```python
from build123d import *

# Parameters (mm, degrees)
SKETCH_1_W           = 300
SKETCH_1_H           = 30
EXTRUDE_1_DEPTH      = 20
EXTRUDE_2_DEPTH      = 28
EXTRUDE_2_DEPTH_BACK = 328
SKETCH_3_R           = 4
CUT_EXTRUDE_1_DEPTH  = 182.614977356
SKETCH_3_3_R         = 6
SKETCH_3_3_R_2       = 4
CUT_EXTRUDE_2_DEPTH  = 182.614977356
SKETCH_3_4_R         = 13.5
SKETCH_3_4_R_2       = 13.25
SKETCH_3_4_R_3       = 6
CUT_EXTRUDE_3_DEPTH  = 182.614977356
SKETCH_3_5_R         = 2.4
CUT_EXTRUDE_4_DEPTH  = 4.5
SKETCH_3_6_R         = 2.4
CUT_EXTRUDE_5_DEPTH  = 5
SKETCH_9_W           = 8.22
SKETCH_9_H           = 5
CUT_EXTRUDE_6_DEPTH  = 182.295339172
CUT_EXTRUDE_7_REACH  = 183.615
SKETCH_11_R          = 2.55


with BuildPart() as part:
    # Sketch 1 → Extrude 1 (new body)
    with BuildSketch(Plane.XY):
        with Locations((0, 15)):
            Rectangle(SKETCH_1_W, SKETCH_1_H)
    extrude(amount=EXTRUDE_1_DEPTH)

    # Sketch 2 → Extrude 2 (add, two sides: drawn at the far end of the back side and taken through both)
    with BuildSketch(Plane.ZY.offset(150).offset(-EXTRUDE_2_DEPTH_BACK)):
        with BuildLine():
            Line((0, 20), (0, 10))
            ThreePointArc((0, 10), (5, 15), (0, 20))
        make_face()
    extrude(amount=EXTRUDE_2_DEPTH + EXTRUDE_2_DEPTH_BACK)

    # Sketch 3 → Cut-Extrude 1 (cut, through all)
    with BuildSketch(Plane(origin=(0, 0, 0), x_dir=(-1, 0, 0), z_dir=(0, 0, -1))):
        with Locations((0, 15)):
            Circle(SKETCH_3_R)
    extrude(amount=-CUT_EXTRUDE_1_DEPTH, mode=Mode.SUBTRACT)

    # Sketch 3_3 → Cut-Extrude 2 (cut, through all)
    with BuildSketch(Plane(origin=(0, 0, 0), x_dir=(-1, 0, 0), z_dir=(0, 0, -1))):
        with Locations((0, 15)):
            Circle(SKETCH_3_3_R)
        with Locations((0, 15)):
            Circle(SKETCH_3_3_R_2, mode=Mode.SUBTRACT)
    extrude(amount=-CUT_EXTRUDE_2_DEPTH, mode=Mode.SUBTRACT)

    # Sketch 3_4 → Cut-Extrude 3 (cut, through all)
    # profile 1 of 2: a face of its own
    with BuildSketch(Plane(origin=(0, 0, 0), x_dir=(-1, 0, 0), z_dir=(0, 0, -1))):
        with Locations((0, 15)):
            Circle(SKETCH_3_4_R)
        with Locations((0, 15)):
            Circle(SKETCH_3_4_R_2, mode=Mode.SUBTRACT)
    # profile 2 of 2: a face of its own
    with BuildSketch(Plane(origin=(0, 0, 0), x_dir=(-1, 0, 0), z_dir=(0, 0, -1))):
        with Locations((0, 15)):
            Circle(SKETCH_3_4_R_2)
        with Locations((0, 15)):
            Circle(SKETCH_3_4_R_3, mode=Mode.SUBTRACT)
    extrude(amount=-CUT_EXTRUDE_3_DEPTH, mode=Mode.SUBTRACT)

    # Sketch 3_5 → Cut-Extrude 4 (cut)
    # profile 1 of 2: a face of its own
    with BuildSketch(Plane(origin=(0, 0, 0), x_dir=(-1, 0, 0), z_dir=(0, 0, -1))):
        with BuildLine():
            ThreePointArc((-6.02027027, 2.916691435), (-13.5, 15), (-6.02027027, 27.083308565))
            Line((-6.02027027, 27.083308565), (-20.841216216, 19.699064442))
            ThreePointArc((-20.841216216, 19.699064442), (-23.75, 15), (-20.841216216, 10.300935558))
            Line((-20.841216216, 10.300935558), (-6.02027027, 2.916691435))
        make_face()
        with Locations((-18.5, 15)):
            Circle(SKETCH_3_5_R, mode=Mode.SUBTRACT)
    # profile 2 of 2: a face of its own
    with BuildSketch(Plane(origin=(0, 0, 0), x_dir=(-1, 0, 0), z_dir=(0, 0, -1))):
        with BuildLine():
            Line((20.841216216, 19.699064442), (6.02027027, 27.083308565))
            ThreePointArc((6.02027027, 27.083308565), (11.478755347, 22.105503197), (13.5, 15))
            ThreePointArc((13.5, 15), (11.478755347, 7.894496803), (6.02027027, 2.916691435))
            Line((6.02027027, 2.916691435), (20.841216216, 10.300935558))
            ThreePointArc((20.841216216, 10.300935558), (23.75, 15), (20.841216216, 19.699064442))
        make_face()
        with Locations((18.5, 15)):
            Circle(SKETCH_3_5_R, mode=Mode.SUBTRACT)
    extrude(amount=-CUT_EXTRUDE_4_DEPTH, mode=Mode.SUBTRACT)

    # Sketch 3_6 → Cut-Extrude 5 (cut)
    with BuildSketch(Plane(origin=(0, 0, 0), x_dir=(-1, 0, 0), z_dir=(0, 0, -1))):
        with Locations((-18.5, 15)):
            Circle(SKETCH_3_6_R)
        with Locations((18.5, 15)):
            Circle(SKETCH_3_6_R)
    extrude(amount=-CUT_EXTRUDE_5_DEPTH, mode=Mode.SUBTRACT)

    # Sketch 6 → Loft 2 section 0
    with BuildSketch(Plane.XZ):
        with BuildLine():
            Line((-143.03, 4), (-130.81, 4))
            Line((-130.81, 4), (-130.81, 9))
            Line((-130.81, 9), (-143.03, 9))
            Line((-143.03, 9), (-143.03, 4))
        make_face()
    # Sketch 7 → Loft 2 section 1
    with BuildSketch(Plane(origin=(0, 2, 0), x_dir=(-1, 0, 0), z_dir=(0, -1, 0))):
        with BuildLine():
            Line((132.81, -9), (141.03, -9))
            Line((141.03, -9), (141.03, -4))
            Line((141.03, -4), (132.81, -4))
            Line((132.81, -4), (132.81, -9))
        make_face()
    loft_2 = loft(mode=Mode.SUBTRACT)

    # Sketch 4 → Loft 3 section 0
    with BuildSketch(Plane(origin=(0, 30, 0), x_dir=(1, 0, 0), z_dir=(0, 1, 0))):
        with BuildLine():
            Line((-143.03, -9), (-130.81, -9))
            Line((-130.81, -9), (-130.81, -4))
            Line((-130.81, -4), (-143.03, -4))
            Line((-143.03, -4), (-143.03, -9))
        make_face()
    # Sketch 5 → Loft 3 section 1
    with BuildSketch(Plane(origin=(0, 28, 0), x_dir=(1, 0, 0), z_dir=(0, 1, 0))):
        with BuildLine():
            Line((-141.03, -9), (-132.81, -9))
            Line((-132.81, -9), (-132.81, -4))
            Line((-132.81, -4), (-141.03, -4))
            Line((-141.03, -4), (-141.03, -9))
        make_face()
    loft_3 = loft(mode=Mode.SUBTRACT)

    # Sketch 9 → Cut-Extrude 6 (cut, through all)
    with BuildSketch(Plane(origin=(0, 28, 0), x_dir=(1, 0, 0), z_dir=(0, 1, 0))):
        with Locations((-136.92, -6.5)):
            Rectangle(SKETCH_9_W, SKETCH_9_H)
    cut_extrude_6 = extrude(amount=-CUT_EXTRUDE_6_DEPTH, mode=Mode.SUBTRACT)

    # Mirror 2: Loft 2, Loft 3, Cut-Extrude 6 across plane
    add(loft_2.mirror(Plane(origin=(0, 0, 0), x_dir=(0, 0, 1), z_dir=(1, 0, 0))), mode=Mode.SUBTRACT)
    add(loft_3.mirror(Plane(origin=(0, 0, 0), x_dir=(0, 0, 1), z_dir=(1, 0, 0))), mode=Mode.SUBTRACT)
    add(cut_extrude_6.mirror(Plane(origin=(0, 0, 0), x_dir=(0, 0, 1), z_dir=(1, 0, 0))), mode=Mode.SUBTRACT)

    # Sketch 11 → Cut-Extrude 7 (cut, up to next)
    with BuildSketch(Plane(origin=(0, 0, 0), x_dir=(-1, 0, 0), z_dir=(0, 0, -1)), mode=Mode.PRIVATE) as cut_extrude_7_sk1:
        with Locations((-136.92, 15)):
            Circle(SKETCH_11_R)
    cut_extrude_7_tool1 = extrude(cut_extrude_7_sk1.sketch, amount=-CUT_EXTRUDE_7_REACH, mode=Mode.PRIVATE) & part.part
    cut_extrude_7 = cut_extrude_7_tool1.solids().sort_by_distance((136.92, 15, 0))[0]
    add(cut_extrude_7, mode=Mode.SUBTRACT)

    # Mirror 3: Cut-Extrude 7 across plane
    add(cut_extrude_7.mirror(Plane(origin=(0, 0, 0), x_dir=(0, 0, 1), z_dir=(1, 0, 0))), mode=Mode.SUBTRACT)


solid = part.part
```
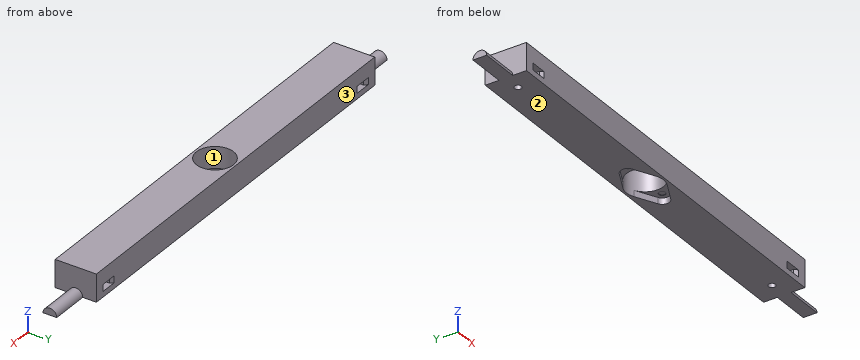
Design review of the part built by this model. Coordinates are the model's own, in mm. Face numbers are marked on the shaded views. Coordinates: 2 decimals unless noted, no trailing zeros. Loops run counter-clockwise (first coordinate to the right, second up) from the corner with the lowest first, then second, coordinate; pieces in that order, holes last. Notation, with made-up numbers: (28, 44) -> (81, 44) arc R25 ccw to (81, 70) -> close; hole circle Ø4 at (-7, -19). An arc over 180 degrees is marked (long way). Answer as a JSON object with one key per item and string values.
Q1. The part is to be moulded in two halves that separate along Y. For the marked faces 1, 2 and 3, say which applies: +Y half, -Y half, draft (parallel to the pull), parting line (faces both ways), or undercut.
Answer block:
{"face 1": "undercut", "face 2": "draft", "face 3": "+Y half"}
Q2. Take a section at A-A on z = 12.5. Give the boundary of the cut face in (x, y), plus the area to 3 significant figures.
Answer block:
{"outline": "(-150, 0) -> (150, 0) -> (150, 30) -> (-150, 30) -> close; hole circle Ø27 at (0, 15)", "area": "8,430 mm^2"}
Q3. Clearance check with flat-ended pins moving along their axes: pin 1 Ø2.5 at (x, y) = (19, 15.5) entering from -Z; pin 2 Ø2.5 at (y, z) = (15, 7.5) entering from +X; pin 3 Ø5.5 at (x, y) = (-18.5, 14.5) entering from -Z. State where each tip first meets the part, or that it passes through.
Answer block:
{"pin 1": "stops at z = 5", "pin 2": "stops at x = 150", "pin 3": "stops at z = 4.5"}
Q4. To check wall thickness, follow L1, parallel to Y at x = 0, z = 14.5; L2, parallel to Y at x = 18.5, z = 4.9; L3, parallel to X at y = 23, z = 6.25. State the ranges of each line that lie inside material, in increasing order.
Answer block:
{"L1": "y = 0 to 1.5, 28.5 to 30", "L2": "y = 0 to 12.6, 17.4 to 30", "L3": "x = -150 to -141.03, -132.81 to -10.87, 10.87 to 132.81, 141.03 to 150"}
